```python
from build123d import *

# Parameters (mm, degrees)
SKETCH1_R                        = 23.01875
BOSS_EXTRUDE1_DEPTH              = 44.45
SKETCH2_R                        = 25.4
BOSS_EXTRUDE2_DEPTH              = 6.35
SKETCH3_R                        = 9.5
CUT_EXTRUDE1_DEPTH               = 63.217039467
SKETCH4_R                        = 16.6751
CUT_EXTRUDE2_DEPTH               = 44.45
SKETCH5_R                        = 1.5875
CUT_EXTRUDE3_DEPTH               = 19.05
TAP_DRILL_FOR_1_4_20_TAP1_REACH  = 76.634
TAP_DRILL_FOR_1_4_20_TAP1_BORE_R = 2.5527


with BuildPart() as part:
    # Sketch1 → Boss-Extrude1 (new body)
    with BuildSketch(Plane(origin=(0, 0, 0), x_dir=(1, 0, 0), z_dir=(0, 1, 0))):
        with Locations(Location((0, 0, 0), (0, 0, 270))):
            Circle(SKETCH1_R)
    extrude(amount=BOSS_EXTRUDE1_DEPTH)

    # Sketch2 → Boss-Extrude2 (add)
    with BuildSketch(Plane(origin=(0, 44.45, 0), x_dir=(1, 0, 0), z_dir=(0, 1, 0))):
        with Locations(Location((0, 0, 0), (0, 0, 270))):
            Circle(SKETCH2_R)
    extrude(amount=BOSS_EXTRUDE2_DEPTH)

    # Sketch3 → Cut-Extrude1 (cut, through all)
    with BuildSketch(Plane(origin=(0, 50.8, 0), x_dir=(1, 0, 0), z_dir=(0, 1, 0))):
        with Locations(Location((0, 0, 0), (0, 0, 270))):
            Circle(SKETCH3_R)
    extrude(amount=-CUT_EXTRUDE1_DEPTH, mode=Mode.SUBTRACT)

    # Sketch4 → Cut-Extrude2 (cut)
    with BuildSketch(Plane.XZ):
        with Locations(Location((0, 0, 0), (0, 0, 270))):
            Circle(SKETCH4_R)
    extrude(amount=-CUT_EXTRUDE2_DEPTH, mode=Mode.SUBTRACT)

    # Sketch5 → Cut-Extrude3 (cut)
    with BuildSketch(Plane.XZ):
        with Locations(Location((19.84375, 0, 0), (0, 0, 270))):
            Circle(SKETCH5_R)
        with Locations(Location((9.921875, -17.185191606, 0), (0, 0, 270))):
            Circle(SKETCH5_R)
        with Locations(Location((-9.921875, -17.185191606, 0), (0, 0, 270))):
            Circle(SKETCH5_R)
        with Locations(Location((-19.84375, 0, 0), (0, 0, 270))):
            Circle(SKETCH5_R)
        with Locations(Location((-9.921875, 17.185191606, 0), (0, 0, 270))):
            Circle(SKETCH5_R)
        with Locations(Location((9.921875, 17.185191606, 0), (0, 0, 270))):
            Circle(SKETCH5_R)
    extrude(amount=-CUT_EXTRUDE3_DEPTH, mode=Mode.SUBTRACT)

    # Tap Drill for 1/4-20 Tap1 bore → Tap Drill for 1/4-20 Tap1 (cut, up to next)
    with BuildSketch(Plane.ZY.offset(23.01875), mode=Mode.PRIVATE) as tap_drill_for_1_4_20_tap1_sk1:
        with Locations((0, 31.75)):
            Circle(TAP_DRILL_FOR_1_4_20_TAP1_BORE_R)
    tap_drill_for_1_4_20_tap1_tool1 = extrude(tap_drill_for_1_4_20_tap1_sk1.sketch, amount=-TAP_DRILL_FOR_1_4_20_TAP1_REACH, mode=Mode.PRIVATE) & part.part
    add(tap_drill_for_1_4_20_tap1_tool1.solids().sort_by_distance((-23.01875, 31.75, 0))[0], mode=Mode.SUBTRACT)


solid = part.part
```
Can you work these out from the model? Positions are in its coordinate system, mm. A direction names the side the tool comes from. Coordinates: 2 decimals unless noted, no trailing zeros. Loops run counter-clockwise (first coordinate to the right, second up) from the corner with the lowest first, then second, coordinate; pieces in that order, holes last. Notation, with made-up numbers: (-2, 48.5) - (6, 48.5) arc R19 cw to (6, 84.5) - close; hole circle Ø6 at (13.5, 3.5). An arc over 180 degrees is marked (long way). Use a Markdown table: item, result.
Item 1: I want a section at C-C on y = 39.5. Please give me the cut outline in (x, z).
Numbers:
| item | result |
|---|---|
| outline | circle Ø46.04 at (0, 0); hole circle Ø33.35 at (0, 0) |
Item 2: For faces 1 (the face through (10, 19.05, -17)), 2 (the face through (-5.78, 47.67, -7.54)), 3 (the face through (-19.795, 29.258, -0.553)), which set-ups out of +Z, -Z, +X, -X, +Y, -Y let a thin tool reach every point of the face, with its end or its side?
Numbers:
| item | result |
|---|---|
| face 1 | -Y |
| face 2 | +Y, -Y |
| face 3 | -X |
Item 3: We'd pull the mould along Z, two halves only. Please class faces 4 (the face through (20, 19.05, 0)), 5 (the face through (0, 50.8, 11)), 6 (the face through (-22.47, 21.91, -4.99)): released by +Z, released by -Z, zero draft, split by the parting line, or undercut.
Numbers:
| item | result |
|---|---|
| face 4 | undercut |
| face 5 | zero draft |
| face 6 | split by the parting line |
Item 4: I want a section at A-A on x = 0. Please give me the cut outline in (y, z).
Numbers:
| item | result |
|---|---|
| outline | (0, -23.02) - (44.45, -23.02) - (44.45, -25.4) - (50.8, -25.4) - (50.8, -9.5) - (44.45, -9.5) - (44.45, -16.68) - (0, -16.68) - close; (0, 16.68) - (44.45, 16.68) - (44.45, 9.5) - (50.8, 9.5) - (50.8, 25.4) - (44.45, 25.4) - (44.45, 23.02) - (0, 23.02) - close |
Item 5: I want a section at B-B on z = 0. Please give me the cut outline in (x, y).
Numbers:
| item | result |
|---|---|
| outline | (-25.4, 44.45) - (-23.02, 44.45) - (-23.02, 34.3) - (-16.68, 34.3) - (-16.68, 44.45) - (-9.5, 44.45) - (-9.5, 50.8) - (-25.4, 50.8) - close; (-23.02, 0) - (-21.43, 0) - (-21.43, 19.05) - (-18.26, 19.05) - (-18.26, 0) - (-16.68, 0) - (-16.68, 29.2) - (-23.02, 29.2) - close; (9.5, 44.45) - (16.68, 44.45) - (16.68, 0) - (18.26, 0) - (18.26, 19.05) - (21.43, 19.05) - (21.43, 0) - (23.02, 0) - (23.02, 44.45) - (25.4, 44.45) - (25.4, 50.8) - (9.5, 50.8) - close |
Item 6: If I drill on probe 1 along Y at (x, z) = (-19.75, 0); probe 2 along X at (y, z) = (47, 0); probe 3 along X at (y, z) = (5, 0), over which ranges is the centre line in solid material (lowest first)? Write a range as from..to.
Numbers:
| item | result |
|---|---|
| probe 1 | y = 19.05..29.2, 34.3..50.8 |
| probe 2 | x = -25.4..-9.5, 9.5..25.4 |
| probe 3 | x = -23.02..-21.43, -18.26..-16.68, 16.68..18.26, 21.43..23.02 |
Item 7: I want a section at D-D on z = -8. Please give me the cut outline in (x, y), and give its area (3 significant figures).
Numbers:
| item | result |
|---|---|
| outline | (-24.11, 44.45) - (-21.58, 44.45) - (-21.58, 0) - (-14.63, 0) - (-14.63, 44.45) - (-5.12, 44.45) - (-5.12, 50.8) - (-24.11, 50.8) - close; (5.12, 44.45) - (14.63, 44.45) - (14.63, 0) - (21.58, 0) - (21.58, 44.45) - (24.11, 44.45) - (24.11, 50.8) - (5.12, 50.8) - close |
| area | 859 mm2 |
Item 8: Will these pins go through, and if not, where does the flat tip stop? pin 1 (8 mm diameter, centred on y = 31.75, z = 0, fed in from -X); pin 2 (6 mm diameter, centred on x = 17.5, y = 26.5, fed in from -Z); pin 3 (10 mm diameter, centred on x = 1.5, z = -0.5, fed in from -Y); pin 4 (1.5 mm diameter, centred on y = 43.5, z = 9, fed in from +X).
Numbers:
| item | result |
|---|---|
| pin 1 | stops at x = -23.02 |
| pin 2 | stops at z = -17.88 |
| pin 3 | passes through |
| pin 4 | stops at x = 21.49 |
